Can you work these out from the drawing? Everything is in mm from the part's minimum corner. A direction names the side the tool comes from. Round coordinates to 2 decimals unless told otherwise and drop trailing zeros. Loops run counter-clockwise (first coordinate to the right, second up) from the corner with the lowest first, then second, coordinate; pieces in that order, holes last. Notation, with made-up numbers: M 49,40 L 57,40 A26 cw 57,57 Z; hole C 2.5,-12.75 d11. An arc over 180 degrees is marked long. Answer in a Markdown table with one row per item.
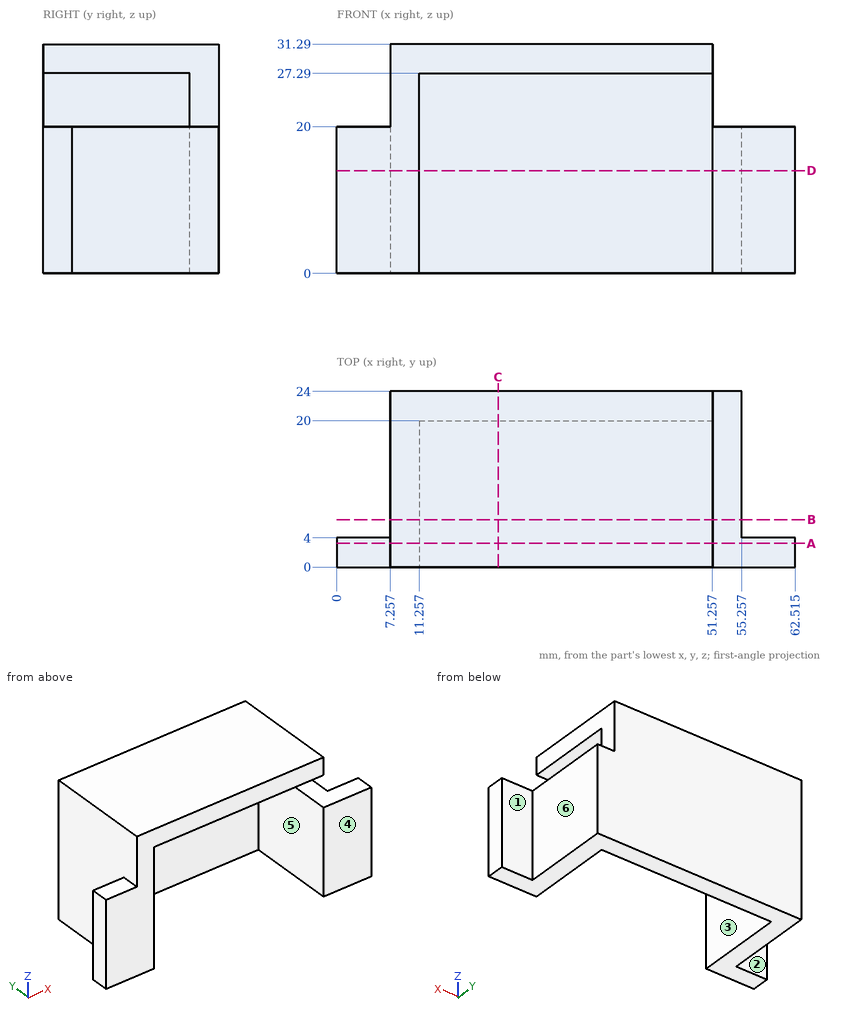
1) I want a section at D-D, the plane z = 14. Please give me the cut outline in (x, y) (1 decimal), plus the area to 3 significant figures.
Computed:
| item | result |
|---|---|
| outline | M 0,0 L 11.3,0 L 11.3,20 L 51.3,20 L 51.3,0 L 62.5,0 L 62.5,4 L 55.3,4 L 55.3,24 L 7.3,24 L 7.3,4 L 0,4 Z |
| area | 410 mm² |
2) If we mould it in two halves opening along X, with no side actions, what happens to the marked faces 4, 5 and 6? For each: released by +X, released by -X, zero draft, split by the parting line, or undercut.
Computed:
| item | result |
|---|---|
| face 4 | zero draft |
| face 5 | undercut |
| face 6 | released by +X |
3) I want a section at A-A, the plane y = 3.25. Please give me the cut outline in (x, z) (1 decimal).
Computed:
| item | result |
|---|---|
| outline | M 0,0 L 11.3,0 L 11.3,27.3 L 51.3,27.3 L 51.3,31.3 L 7.3,31.3 L 7.3,20 L 0,20 Z; M 51.3,0 L 62.5,0 L 62.5,20 L 51.3,20 Z |
4) I want a section at C-C, the plane x = 22. Please give me the cut outline in (y, z), plus the area to 3 significant figures.
Computed:
| item | result |
|---|---|
| outline | M 0,27.29 L 20,27.29 L 20,0 L 24,0 L 24,31.29 L 0,31.29 Z |
| area | 205 mm² |
5) Which directions (+Z, -Z, +X, -X, +Y, -Y) give clear straight access to the entire face, cutting with the end or side of a thin tool? Please do the marked faces 1, 2 and 3.
Computed:
| item | result |
|---|---|
| face 1 | +Z, -Z, +X, +Y |
| face 2 | +Z, -Z, -X, +Y |
| face 3 | -Z, -Y |
6) I want a section at B-B, the plane y = 6.5. Please give me the cut outline in (x, z).
Computed:
| item | result |
|---|---|
| outline | M 7.26,0 L 11.26,0 L 11.26,27.29 L 51.26,27.29 L 51.26,31.29 L 7.26,31.29 Z; M 51.26,0 L 55.26,0 L 55.26,20 L 51.26,20 Z |
7) I need wall thicknesses on line 1 (X direction, y = 15.25, z = 5); line 2 (X direction, y = 2, z = 7) (1 decimal); line 3 (Z direction, x = 21.5, y = 15). Which ranges of each line are inside material? Lowest first, please.
Computed:
| item | result |
|---|---|
| line 1 | x = 7.26 to 11.26, 51.26 to 55.26 |
| line 2 | x = 0 to 11.3, 51.3 to 62.5 |
| line 3 | z = 27.29 to 31.29 |
8) Will these pins go through, and if not, where does the flat tip stop? P1, Ø2, axis at x = 2, z = 6.5, coming from the +Y side; P2, Ø3, axis at x = 18.5, z = 19.5, coming from the -Y side; P3, Ø12, axis at y = 20, z = 12, coming from the +X side; P4, Ø1.5, axis at x = 28, y = 20, coming from the -Z side.
Computed:
| item | result |
|---|---|
| P1 | stops at y = 4 |
| P2 | stops at y = 20 |
| P3 | stops at x = 55.26 |
| P4 | stops at z = 0 |
